Autodesk Inventor part; units mm, degrees
ref_plane "YZ Plane" through (0, 0, 0) normal (1, 0, 0) x (0, 1, 0)
ref_plane "XZ Plane" through (0, 0, 0) normal (0, 1, 0) x (-1, 0, 0)
ref_plane "XY Plane" through (0, 0, 0) normal (0, 0, 1) x (1, 0, 0)
sketch "スケッチ1" plane through (0, 0, 0) normal (0, 0, 1) x (1, 0, 0)
  circle A0 centre (21.005288, 4.842186) radius 2
  circle A1 centre (0, 0) radius 2
  circle A2 centre (81.171801, -23.481667) radius 63
  arc A3 (-1.921226, 0.555779) -> (4.088443, -62.729672) centre (81.171801, -23.481667) ccw
  line L0 (0, 2) -> (9.827028, 2)
  line L1 (11.368602, 2.725814) -> (16.319283, 8.715397)
  line L2 (19.135043, 8.982785) -> (29.075493, 0.766521)
  line L3 (8.206239, 4.393532) -> (1.777293, 9.707368)
  line L4 (40.328272, 40.117124) -> (11.021999, 4.660921)
  arc A4 (9.827028, 2) -> (11.368602, 2.725814) centre (9.827028, 4) ccw
  arc A5 (19.135043, 8.982785) -> (16.319283, 8.715397) centre (17.860857, 7.441211) ccw
  arc A6 (29.641669, -1.55804) -> (34.689305, -54.712702) centre (81.171801, -23.481667) ccw
  circle A7 centre (5.870717, -61.822204) radius 2
  circle A8 centre (27.411976, -62.624114) radius 2
  line L5 (81.171801, -23.481667) -> (18.171801, -23.481667)
  line L6 (34.57079, -57.102281) -> (26.354526, -67.042731)
  line L7 (17.573011, -64.325196) -> (53.029214, -93.631469)
  line L8 (17.573011, -64.325196) -> (53.029214, -93.631469)
  line L9 (9.443415, -71.02153) -> (14.757251, -64.592584)
  line L10 (23.538766, -67.310119) -> (17.549183, -62.359438)
  arc A9 (23.538766, -67.310119) -> (26.354526, -67.042731) centre (24.812952, -65.768545) ccw
  line L11 (15.898547, -61.93676) -> (6.247168, -63.786456)
  arc A10 (17.549183, -62.359438) -> (15.898547, -61.93676) centre (16.274997, -63.901012) ccw
  arc A11 (29.641669, -1.55804) -> (29.075493, 0.766521) centre (27.801307, -0.775053) ccw
  arc A12 (34.57079, -57.102281) -> (34.689305, -54.712702) centre (33.029216, -55.828096) ccw
  circle A13 centre (5.870717, -61.822204) radius 1
  circle A14 centre (27.411976, -62.624114) radius 1
  circle A15 centre (21.005288, 4.842186) radius 1
  circle A16 centre (0, 0) radius 1
  point P0 (0, 0)
  point P1 (30.241928, -0.197595)
  point P2 (35.534905, -55.935846)
  dimension "d0" = 1.5
  dimension "d1" = 2
  dimension "d3" = 56
  dimension "d8" = 2
  dimension "d9" = 2
extrude "押し出し1" add sketch "スケッチ1" along normal blind 1.2 contours A0 | A8 | L2 A2 L6 A9 L10 A10 L11 A7 A3 A1 L0 A4 L1 A5 | L2 A11 A6 L5 A2 | L5 A6 A12 L6 A2 | A1 | A7
properties part number "MainMCU_PCB"
The listing builds one solid part. Answer for the finished solid, in the listing's coordinates (mm). A direction names the side the tool comes from. Round coordinates to 2 decimals unless told otherwise and drop trailing zeros. Loops run counter-clockwise (first coordinate to the right, second up) from the corner with the lowest first, then second, coordinate; pieces in that order, holes last. Notation, with made-up numbers: (5, 24.5) - (43, 24.5) arc R22 ccw to (43, 52.5) - close; hole circle Ø1 at (41, 75). An arc over 180 degrees is marked (long way). Return JSON: item names as keys, results as strings. Group by question number.
1. Which of the six approach directions +Z, -Z, +X, -X, +Y, -Y give full straight-line access (tool end or side, diameter ignored) to faces 1 (the flat face through (11.14, -62.85, 0.59)), 2 (the cylindrical face through (27.195, -61.648, 0.592))?
2. This flat-tipped pin is pushed along its axis until it touches: P1, Ø3, axis at x = 21.01, y = 4.84, coming from the -Z side. Where does it stop, or does it pass through?
3. The part is cut by section A-A on z = 0.6. Determine the outline of the cut face in (x, y) (1 decimal).
4. Consider probe 1 along X at (y, z) = (5, 1); probe 2 along Y at (x, z) = (16.5, 0.5); probe 3 along X at (y, z) = (-39.5, 0.25). Determine where each line is inside the solid, lowest interval first.
5. The part is cut by section C-C on x = 2.5. Determine the outline of the cut face in (y, z), then the cut area to 3 significant figures.
6. The part is cut by section B-B on y = -5. Determine the outline of the cut face in (x, z).
7. The mould has two halves that part along X. Classify faces 3 (the cylindrical face through (-1.2, 1.6, 0.6)), 4 (the flat face through (20.586, -64.869, 0.592)), 5 (the flat face through (24.04, 4.93, 0.59)): pulls with the +X half, pulls with the -X half, needs draft (parallel to the pull), parting line crosses it, or undercut.
Resolved:
{
 "1": {"face 1": "+Z, -Z, -Y", "face 2": "+Z, -Z"},
 "2": {"P1": "stops at z = 0"},
 "3": {"outline": "(-1.9, 0.6) arc R86.5 ccw to (4.1, -62.7) arc R2 ccw to (6.2, -63.8) - (15.9, -61.9) arc R2 cw to (17.5, -62.4) - (23.5, -67.3) arc R2 ccw to (26.4, -67) - (34.6, -57.1) arc R2 ccw to (34.7, -54.7) arc R56 cw to (29.6, -1.6) arc R2 ccw to (29.1, 0.8) - (19.1, 9) arc R2 ccw to (16.3, 8.7) - (11.4, 2.7) arc R2 cw to (9.8, 2) - (0, 2) arc R2 ccw to start; hole circle Ø2 at (0, 0); hole circle Ø2 at (5.9, -61.8); hole circle Ø2 at (21, 4.8); hole circle Ø2 at (27.4, -62.6)"},
 "4": {"probe 1": "x = 13.25 to 20.02, 21.99 to 23.95", "probe 2": "y = -61.91 to 8.91", "probe 3": "x = -3.83 to 27.51"},
 "5": {"outline": "(-59.44, 0) - (2, 0) - (2, 1.2) - (-59.44, 1.2) - close", "area": "73.7 mm²"},
 "6": {"outline": "(-3.33, 0) - (28.31, 0) - (28.31, 1.2) - (-3.33, 1.2) - close"},
 "7": {"face 3": "pulls with the -X half", "face 4": "undercut", "face 5": "pulls with the +X half"}
}
